Autodesk Inventor part; units mm, degrees
ref_plane "YZ Plane" through (0, 0, 0) normal (1, 0, 0) x (0, 1, 0)
ref_plane "XZ Plane" through (0, 0, 0) normal (0, 1, 0) x (-1, 0, 0)
ref_plane "XY Plane" through (0, 0, 0) normal (0, 0, 1) x (1, 0, 0)
sketch "Náčrt1" plane through (0, 0, 0) normal (0, 1, 0) x (-1, 0, 0)
  circle A0 centre (0, 0) radius 3.4925
  dimension "d0" = 6.985
extrude "Vysunutí1" add sketch "Náčrt1" along normal blind 8.255
chamfer "Zkosení1" distance 0.3175 distance2 8.255 1 edges at (3.4925, 8.255, 0) measured on face at (-1.152, 8.255, -0.772)
sketch "Náčrt2" plane through (0, 0, 0) normal (0, -1, 0) x (1, 0, 0)
  circle A0 centre (0, 0) radius 3.4925
  line L0 (1.905, -1.905) -> (-1.905, 1.905) construction
  line L1 (-1.905, -1.905) -> (1.905, 1.905) construction
  line L2 (-0.635, 1.905) -> (-0.635, 1.27)
  line L3 (-0.635, 1.27) -> (0.635, 1.27)
  line L4 (0.635, 1.27) -> (0.635, 1.905)
  line L5 (-0.635, -1.905) -> (-0.635, -1.2721)
  line L6 (-0.635, -1.2721) -> (0.635, -1.2721)
  line L7 (0.635, -1.2721) -> (0.635, -1.905)
  line L8 (-1.905, -0.6371) -> (-1.2679, -0.6371)
  line L9 (-1.2679, -0.6371) -> (-1.2679, 0.6371)
  line L10 (-1.2679, 0.6371) -> (-1.905, 0.6371)
  line L11 (1.905, -0.6371) -> (1.2679, -0.6371)
  line L12 (1.2679, -0.6371) -> (1.2679, 0.6371)
  line L13 (1.2679, 0.6371) -> (1.905, 0.6371)
  line L14 (-1.905, -1.905) -> (-1.905, -0.6371)
  line L15 (-1.905, 0.6371) -> (-1.905, 1.905)
  line L16 (-1.905, 1.905) -> (-0.635, 1.905)
  line L17 (0.635, 1.905) -> (1.905, 1.905)
  line L18 (1.905, -1.905) -> (0.635, -1.905)
  line L19 (-0.635, -1.905) -> (-1.905, -1.905)
  line L20 (1.905, 1.905) -> (1.905, 0.6371)
  line L21 (1.905, -0.6371) -> (1.905, -1.905)
  dimension "d6" = 3.81
  dimension "d7" = 3.81
extrude "Vysunutí2" cut sketch "Náčrt2" against normal blind 7.62 contours L2 L3 L4 L17 L20 L13 L12 L11 L21 L18 L7 L6 L5 L19 L14 L8 L9 L10 L15 L16
fillet "Zaoblení1" radius 0.254 1 edges at (3.1755, 8.255, 0)
properties part number "2P1-2TB-B201A-Z_button_circle"
Read the model definition and answer for the solid it produces. Units are mm, in the model's axes. A direction names the side the tool comes from. Coordinates: 2 decimals unless noted, no trailing zeros. Write each loop counter-clockwise with the first axis right and the second up, starting at its lowest first coordinate (ties: lowest second). Pieces come first, ordered by that corner, then holes. Notation, with made-up numbers: M 64.5,28.5 L 71.5,28.5 A8 ccw 71.5,43.5 Z; hole C 54.5,3.5 d8. An arc over 180 degrees is marked long. Use a Markdown table: item, result.
Q1. The part is cut by section D-D, the plane y = 3. Write down the section's boundary in (x, z) (3 decimals).
Answer block:
| item | result |
|---|---|
| outline | C 0,0 d6.755; hole M -1.905,-1.905 L -0.635,-1.905 L -0.635,-1.272 L 0.635,-1.272 L 0.635,-1.905 L 1.905,-1.905 L 1.905,-0.637 L 1.268,-0.637 L 1.268,0.637 L 1.905,0.637 L 1.905,1.905 L 0.635,1.905 L 0.635,1.27 L -0.635,1.27 L -0.635,1.905 L -1.905,1.905 L -1.905,0.637 L -1.268,0.637 L -1.268,-0.637 L -1.905,-0.637 Z |
Q2. Which of the six approach directions +Z, -Z, +X, -X, +Y, -Y give full straight-line access (tool end or side, diameter ignored) to faces 4 (the face through (-1, 4, 1.905)), 5 (the face through (-2, 0, 0))?
Answer block:
| item | result |
|---|---|
| face 4 | -Y |
| face 5 | +Z, -Z, +X, -X, -Y |
Q3. The part is cut by section C-C, the plane y = 0.5. Write down the section's boundary in (x, z) (3 decimals), then the cut area to 3 significant figures.
Answer block:
| item | result |
|---|---|
| outline | C 0,0 d6.947; hole M -1.905,-1.905 L -0.635,-1.905 L -0.635,-1.272 L 0.635,-1.272 L 0.635,-1.905 L 1.905,-1.905 L 1.905,-0.637 L 1.268,-0.637 L 1.268,0.637 L 1.905,0.637 L 1.905,1.905 L 0.635,1.905 L 0.635,1.27 L -0.635,1.27 L -0.635,1.905 L -1.905,1.905 L -1.905,0.637 L -1.268,0.637 L -1.268,-0.637 L -1.905,-0.637 Z |
| area | 26.6 mm2 |
Q4. Straight lines are drawn through the part: L1, parallel to Z at x = -1.75, y = 2 (3 decimals); L2, parallel to Z at x = 1.75, y = 4.75 (3 decimals); L3, parallel to X at y = 4, z = 1.75 (3 decimals). For each, find the intervals that lie inside material, in ascending order. Write a range as [from, to].
Answer block:
| item | result |
|---|---|
| L1 | z = [-2.933, -1.905], [-0.637, 0.637], [1.905, 2.933] |
| L2 | z = [-2.81, -1.905], [-0.637, 0.637], [1.905, 2.81] |
| L3 | x = [-2.844, -1.905], [-0.635, 0.635], [1.905, 2.844] |
Q5. Determine the mould class of faces 1 (the face through (0, 8.255, 0)), 2 (the face through (2.651, 3.95, 2.033)), 3 (the face through (1, 4, -1.905)) for opening direction X: released by +X, released by -X, zero draft, split by the parting line, or undercut.
Answer block:
| item | result |
|---|---|
| face 1 | zero draft |
| face 2 | split by the parting line |
| face 3 | undercut |
Q6. Each of these flat-tipped pins is pushed along its axis until it touches: pin 1 Ø4 at (y, z) = (6, 2.5) entering from +X; pin 2 Ø1.4 at (y, z) = (5.5, 0.5) entering from -X; pin 3 Ø0.6 at (y, z) = (5.5, 0) entering from +X. Where does it stop, or does it pass through?
Answer block:
| item | result |
|---|---|
| pin 1 | stops at x = 3.23 |
| pin 2 | stops at x = -3.3 |
| pin 3 | stops at x = 3.29 |
